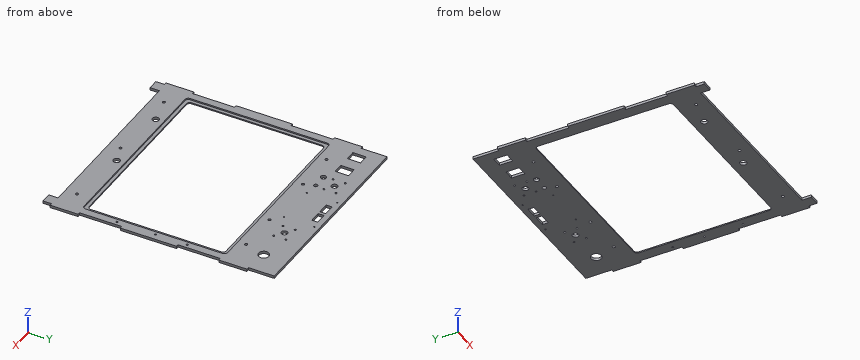
Autodesk Inventor part; units mm, degrees
ref_plane "YZ Plane" through (0, 0, 0) normal (1, 0, 0) x (0, 1, 0)
ref_plane "XZ Plane" through (0, 0, 0) normal (0, 1, 0) x (-1, 0, 0)
ref_plane "XY Plane" through (0, 0, 0) normal (0, 0, 1) x (1, 0, 0)
sketch "Sketch1" plane through (0, 0, 0) normal (0, 0, 1) x (1, 0, 0)
  line L0 (67.9652, 2.3975) -> (457.9652, 2.3975)
  line L1 (479.9652, -17.6025) -> (457.9652, -17.6025)
  line L2 (457.9652, -17.6025) -> (457.9652, 2.3975)
  line L3 (45.9652, -17.6025) -> (67.9652, -17.6025)
  line L4 (67.9652, -17.6025) -> (67.9652, 2.3975)
  line L5 (479.9652, 59.8925) -> (479.9652, 59.8925)
  line L6 (456.9652, 57.3975) -> (68.9652, 57.3975)
  line L7 (36.9652, 522.3965) -> (36.9552, 522.3965)
  line L8 (463.9652, 64.3975) -> (463.9652, 356.3975)
  line L9 (61.9652, 64.3975) -> (61.9652, 356.3975)
  line L10 (68.9652, 363.3975) -> (456.9652, 363.3975)
  line L11 (479.9652, 150.3975) -> (485.4652, 150.3975)
  line L12 (479.9652, 270.3975) -> (485.4652, 270.3975)
  line L13 (485.4652, 270.3975) -> (485.4652, 150.3975)
  line L14 (40.4652, 270.3975) -> (40.4652, 150.3975)
  line L15 (40.4652, 150.3975) -> (45.9652, 150.3975)
  line L16 (40.4652, 270.3975) -> (45.9652, 270.3975)
  circle A0 centre (95.9652, 27.3975) radius 3
  circle A1 centre (429.9652, 27.3975) radius 3
  circle A2 centre (417.4652, 381.0395) radius 3
  circle A3 centre (108.4652, 381.0395) radius 3
  circle A4 centre (327.4652, 381.0395) radius 3
  circle A5 centre (198.4652, 381.0395) radius 3
  circle A6 centre (262.9652, 27.3975) radius 3
  circle A7 centre (471.4652, 135.3975) radius 2
  circle A8 centre (471.4652, 285.3975) radius 2
  line L17 (45.9652, 270.3975) -> (45.9652, 360.3975)
  line L18 (45.9652, 360.3975) -> (40.4652, 360.3975)
  line L19 (40.4652, 360.3975) -> (40.4652, 420.3975)
  line L20 (40.4652, 420.3975) -> (45.9652, 420.3975)
  line L21 (45.9652, 475.4975) -> (45.9652, 420.3975)
  line L22 (45.9652, 360.3975) -> (45.9652, 270.3975)
  line L23 (45.9652, 150.3975) -> (45.9652, 60.3975)
  line L24 (45.9652, 60.3975) -> (40.4652, 60.3975)
  line L25 (40.4652, 60.3975) -> (40.4652, 0.3975)
  line L26 (40.4652, 0.3975) -> (45.9652, 0.3975)
  line L27 (45.9652, 150.3975) -> (45.9652, 60.3975)
  line L28 (45.9652, 0.3975) -> (45.9652, -17.6025)
  line L29 (479.9652, 360.3975) -> (485.4652, 360.3975)
  line L30 (485.4652, 360.3975) -> (485.4652, 420.3975)
  line L31 (485.4652, 420.3975) -> (479.9652, 420.3975)
  line L32 (479.9652, 475.4975) -> (479.9652, 420.3975)
  line L33 (479.9652, 150.3975) -> (479.9652, 60.3975)
  line L34 (479.9652, 60.3975) -> (485.4652, 60.3975)
  line L35 (485.4652, 60.3975) -> (485.4652, 0.3975)
  line L36 (485.4652, 0.3975) -> (479.9652, 0.3975)
  line L37 (479.9652, -17.6025) -> (479.9652, 0.3975)
  line L38 (479.9652, 60.3975) -> (479.9652, 150.3975)
  line L39 (479.9652, 270.3975) -> (479.9652, 360.3975)
  line L40 (262.9652, 474.8975) -> (262.9652, 460.6682)
  circle A9 centre (218.9652, 465.4975) radius 1.5
  circle A10 centre (218.9652, 400.4975) radius 1.5
  circle A11 centre (306.9652, 465.4975) radius 1.5
  circle A12 centre (306.9652, 400.4975) radius 1.5
  line L41 (266.4652, 463.3975) -> (290.7652, 463.3975)
  line L42 (290.7652, 463.3975) -> (290.7652, 450.7975)
  line L43 (290.7652, 450.7975) -> (266.4652, 450.7975)
  line L44 (266.4652, 450.7975) -> (266.4652, 463.3975)
  line L45 (235.4652, 463.3975) -> (259.7652, 463.3975)
  line L46 (259.7652, 463.3975) -> (259.7652, 450.7975)
  line L47 (259.7652, 450.7975) -> (235.4652, 450.7975)
  line L48 (235.4652, 450.7975) -> (235.4652, 463.3975)
  line L49 (86.9652, 440.4975) -> (65.4652, 440.4975)
  line L50 (65.4652, 440.4975) -> (65.4652, 414.9975)
  line L51 (65.4652, 414.9975) -> (86.9652, 414.9975)
  line L52 (86.9652, 414.9975) -> (86.9652, 440.4975)
  line L53 (87.0652, 441.9975) -> (87.0652, 413.4975)
  line L54 (65.3652, 413.4975) -> (65.3652, 441.9975)
  line L55 (133.4652, 440.4975) -> (111.9652, 440.4975)
  line L56 (111.9652, 440.4975) -> (111.9652, 414.9975)
  line L57 (111.9652, 414.9975) -> (133.4652, 414.9975)
  line L58 (133.4652, 414.9975) -> (133.4652, 440.4975)
  line L59 (133.5652, 441.9975) -> (133.5652, 413.4975)
  line L60 (111.8652, 413.4975) -> (111.8652, 441.9975)
  circle A13 centre (160.4652, 403.4975) radius 6
  circle A14 centre (175.4652, 435.4975) radius 6.5
  circle A15 centre (350.4652, 425.4975) radius 6.5
  circle A16 centre (193.4652, 448.4975) radius 2
  circle A17 centre (193.4652, 422.4975) radius 2
  circle A18 centre (157.4652, 448.4975) radius 2
  circle A19 centre (157.4652, 422.4975) radius 2
  circle A20 centre (368.4652, 438.4975) radius 2
  circle A21 centre (368.4652, 412.4975) radius 2
  circle A22 centre (332.4652, 438.4975) radius 2
  circle A23 centre (332.4652, 412.4975) radius 2
  circle A24 centre (429.9652, 425.4975) radius 11
  circle A25 centre (190.4652, 403.4975) radius 4.125
  line L61 (45.9652, 475.4975) -> (479.9652, 475.4975)
  line L62 (65.3652, 441.9975) -> (87.0652, 441.9975)
  line L63 (65.3652, 413.4975) -> (87.0652, 413.4975)
  line L64 (111.8652, 441.9975) -> (133.5652, 441.9975)
  line L65 (111.8652, 413.4975) -> (133.5652, 413.4975)
  arc A26 (68.9652, 363.3975) -> (61.9652, 356.3975) centre (68.9652, 356.3975) ccw
  arc A27 (61.9652, 64.3975) -> (68.9652, 57.3975) centre (68.9652, 64.3975) ccw
  arc A28 (456.9652, 57.3975) -> (463.9652, 64.3975) centre (456.9652, 64.3975) ccw
  arc A29 (463.9652, 356.3975) -> (456.9652, 363.3975) centre (456.9652, 356.3975) ccw
  line L66 (449.9652, 356.3975) -> (75.9652, 356.3975)
  line L67 (68.9652, 349.3975) -> (68.9652, 71.3975)
  line L68 (75.9652, 64.3975) -> (449.9652, 64.3975)
  line L69 (456.9652, 71.3975) -> (456.9652, 349.3975)
  arc A30 (75.9652, 356.3975) -> (68.9652, 349.3975) centre (75.9652, 349.3975) ccw
  arc A31 (456.9652, 349.3975) -> (449.9652, 356.3975) centre (449.9652, 349.3975) ccw
  arc A32 (449.9652, 64.3975) -> (456.9652, 71.3975) centre (449.9652, 71.3975) ccw
  arc A33 (68.9652, 71.3975) -> (75.9652, 64.3975) centre (75.9652, 71.3975) ccw
  circle A34 centre (471.4652, 217.4975) radius 2
  point P0 (77.9853, 6.3978)
  point P1 (463.9652, 475.4975)
  dimension "d148" = 55
  dimension "d187" = 434
  dimension "d211" = 168
  dimension "d212" = 5.5
  dimension "d214" = 5.5
  dimension "d218" = 120
  dimension "d220" = 6
  dimension "d229" = 6
  dimension "d234" = 6
  dimension "d235" = 6
  dimension "d238" = 6
  dimension "d239" = 6
  dimension "d243" = 4
  dimension "d245" = 4
  dimension "d247" = 150
  dimension "d248" = 153
  dimension "d254" = 90
  dimension "d256" = 90
  dimension "d257" = 90
  dimension "d258" = 60
  dimension "d259" = 90
  dimension "d260" = 5.5
  dimension "d261" = 60
  dimension "d262" = 90
  dimension "d263" = 5.5
  dimension "d264" = 60
  dimension "d265" = 90
  dimension "d266" = 60
  dimension "d267" = 120
  dimension "d270" = 3
  dimension "d271" = 44
  dimension "d273" = 3
  dimension "d274" = 65
  dimension "d275" = 88
  dimension "d283" = 24.3
  dimension "d284" = 3.5
  dimension "d285" = 24.3
  dimension "d286" = 3.2
  dimension "d288" = 12.6
  dimension "d289" = 12.6
  dimension "d290" = 68
  dimension "d291" = 68
  dimension "d298" = 25
  dimension "d299" = 21.5
  dimension "d300" = 25.5
  dimension "d302" = 21.5
  dimension "d303" = 25.5
  dimension "d305" = 25
  dimension "d307" = 12
  dimension "d311" = 13
  dimension "d333" = 22
  dimension "d334" = 22
  dimension "d437" = 13
  dimension "d440" = 4
  dimension "d441" = 13
  dimension "d442" = 4
  dimension "d444" = 18
  dimension "d445" = 4
  dimension "d446" = 18
  dimension "d447" = 4
  dimension "d448" = 13
  dimension "d449" = 18
  dimension "d450" = 4
  dimension "d451" = 4
extrude "Extrusion6" add sketch "Sketch1" along normal blind 5.5 contours L4 L3 L28 L26 L25 L24 L23 L15 L14 L16 L17 L18 L19 L20 L21 L61 L32 L31 L30 L29 L39 L12 L13 L11 L33 L34 L35 L36 L37 L1 L2 L0
extrude "Extrusión9" add sketch "Sketch1" along normal blind 2.5 contours L6 A27 L9 A26 L10 A29 L8 A28
sketch "Boceto2" plane through (0, 0, 5.5) normal (0, 0, 1) x (1, 0, 0)
  line L0 (67.9652, 2.3975) -> (457.9652, 2.3975)
  circle A0 centre (150.9652, 40.3975) radius 7
  circle A1 centre (300.9652, 40.3975) radius 7
  line L1 (45.9652, 150.3975) -> (45.9652, 60.3975)
  line L2 (45.9652, 60.3975) -> (45.9652, 2.3975)
  dimension "d159" = 14
  dimension "d162" = 14
  dimension "d165" = 150
  dimension "d269" = 105
extrude "Extrusión10" cut sketch "Boceto2" against normal blind 9
properties part number "Frente Carcasa" material "MDF Medium Density Fiberboard"
Verification items for the finished model (mm, model axes). Coordinates: 2 decimals unless noted, no trailing zeros. Order: outer loops, then holes, each group sorted by start corner. A loop starts at its lowest first (then second) coordinate and runs counter-clockwise, first axis right, second up. Notation, with made-up numbers: (62.25, 38) -> (88.25, 38) arc R36 ccw to (88.25, 74) -> close; hole circle Ø10 at (0.5, 77.5). An arc over 180 degrees is marked (long way). Put each result on its own line as item: value. Start each with the question number.
1) Go/stop test with flat-tipped pins: pin 1 (8.5 mm diameter, centred on x = 300.97, y = 40.4, fed in from +Z); pin 2 (3 mm diameter, centred on x = 483.5, z = 2.5, fed in from -Y); pin 3 (1.6 mm diameter, centred on y = -12, z = 3, fed in from +X); pin 4 (1.6 mm diameter, centred on x = 73.5, z = 2.5, fed in from -Y). Record where each tip stops, or that it passes through.
2) Cross-section at A-A (y = 165). Enter the section's corners in (x, z).
3) Cross-section at B-B (x = 397). Enter the section's corners in (y, z), plus the area to 3 significant figures.
4) Material ranges on L1, parallel to Y at x = 126.5, z = 1.35; L2, parallel to Y at x = 276.5, z = 2.75; L3, parallel to X at y = 345, z = 3.2, recorded low to high.
5) Cross-section at C-C (z = 1.25). State how many separate pieces and enclosed holes the cut face has, plus the area to 3 significant figures.
Geometry check:
1. pin 1: passes through
1. pin 2: stops at y = 0.4
1. pin 3: stops at x = 479.97
1. pin 4: stops at y = 2.4
2. outline: (40.47, 0) -> (68.97, 0) -> (68.97, 2.5) -> (61.97, 2.5) -> (61.97, 5.5) -> (40.47, 5.5) -> close; (456.97, 0) -> (485.47, 0) -> (485.47, 5.5) -> (463.97, 5.5) -> (463.97, 2.5) -> (456.97, 2.5) -> close
3. outline: (2.4, 0) -> (64.4, 0) -> (64.4, 2.5) -> (57.4, 2.5) -> (57.4, 5.5) -> (2.4, 5.5) -> close; (356.4, 0) -> (475.5, 0) -> (475.5, 5.5) -> (363.4, 5.5) -> (363.4, 2.5) -> (356.4, 2.5) -> close
3. area: 954 mm^2
4. L1: y = 2.4 to 64.4, 356.4 to 413.5, 442 to 475.5
4. L2: y = 2.4 to 57.4, 363.4 to 450.8, 463.4 to 475.5
4. L3: x = 45.97 to 61.97, 463.97 to 479.97
5. separate pieces: 1
5. enclosed holes: 34
5. area: 92,300 mm^2
